Geometry check sheet. Reference: the model listing, model coordinates, mm. Face numbers are marked on the shaded views. A direction names the side the tool comes from. Give positions to 0.01 mm unless a question says otherwise; leave off trailing zeros. Write each loop counter-clockwise with the first axis right and the second up, starting at its lowest first coordinate (ties: lowest second). Pieces come first, ordered by that corner, then holes.
(1) Mould release check, pull along Z, two halves, no side actions. Record for the marked faces 1, 2 and 3: +Z half, -Z half, draft (parallel to the pull), parting line (faces both ways), or undercut.
(2) Cross-section at C-C (z = 3.75). Record the boundary of the cut face in (x, y), and give its area (3 significant figures).
(3) Cross-section at A-A (x = 0). Record the boundary of the cut face in (y, z).
(4) Cross-section at D-D (y = 6.25). Record the boundary of the cut face in (x, z), and give its area (3 significant figures).
(5) Thickness scan on line 1 along X through (y, z) = (2, 4.75); line 2 along Z through (x, y) = (8.75, 3.5); line 3 along X through (y, z) = (5, 4.5). Record the ranges inside material, lowest first.
(6) Cross-section at B-B (z = 0). Record the boundary of the cut face in (x, y).
(7) Tool access check on the marked faces 4 and 5. Record the directions out of +Z, -Z, +X, -X, +Y, -Y that give a thin tool (end or side, any length) a straight path to the whole face; none if there is none.
(8) Depth check by flat-ended pin: P1, Ø3.5, axis at x = 0, z = -9.525, coming from the +Y side; P2, Ø2, axis at y = 3, z = -8.5, coming from the +X side; P3, Ø4, axis at x = -9, y = 6.5, coming from the -Z side. Enter the tip coordinate at first touch or a pass-through.
```python
from build123d import *

# Parameters (mm, degrees)
SKETCH2_R          = 1.4224
CUT_EXTRUDE1_DEPTH = 21.154223776
CIRPATTERN1_COUNT  = 6


with BuildPart() as part:
    # Sketch1 → Revolve1 (revolve)
    with BuildSketch(Plane.XY, mode=Mode.PRIVATE) as revolve1_sk:
        Polygon((2.9972, 0), (12.7, 0), (12.7, 5.08), (6.096, 5.08), (6.096, 9.144), (2.9972, 9.144), align=None)
    revolve(revolve1_sk.sketch.rotate(Axis((0, 0, 0), (0, 1, 0)), 90), axis=Axis((0, 0, 0), (0, 1, 0)))

    # Sketch2 → Cut-Extrude1 (cut, through all)
    with BuildSketch(Plane(origin=(0, 0, 0), x_dir=(1, 0, 0), z_dir=(0, 1, 0))):
        with Locations(Location((0, 9.525, 0), (0, 0, 270))):
            Circle(SKETCH2_R)
    cut_extrude1 = extrude(amount=CUT_EXTRUDE1_DEPTH, mode=Mode.SUBTRACT)

    # CirPattern1: Cut-Extrude1 ×6 about axis
    cirpattern1_axis = Axis((0, 0, 0), (0, 1, 0))
    for i in range(1, CIRPATTERN1_COUNT):
        add(cut_extrude1.rotate(cirpattern1_axis, i * 360 / CIRPATTERN1_COUNT), mode=Mode.SUBTRACT)


solid = part.part
```
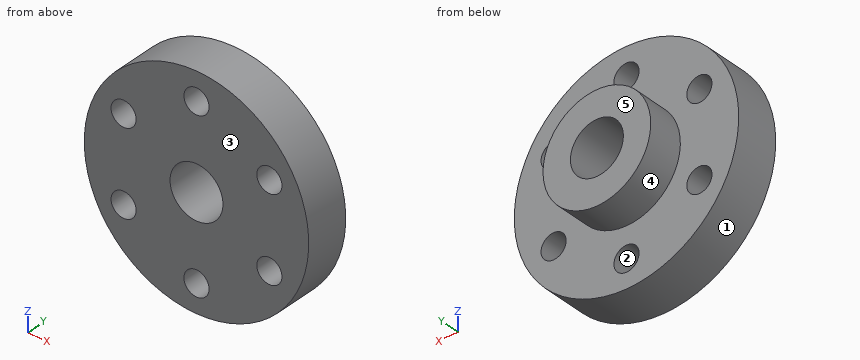
Reply:
1. face 1: parting line
1. face 2: undercut
1. face 3: draft
2. outline: (-12.13, 0) - (-9.25, 0) - (-9.25, 5.08) - (-12.13, 5.08) - close; (-7.25, 0) - (7.25, 0) - (7.25, 5.08) - (4.81, 5.08) - (4.81, 9.14) - (-4.81, 9.14) - (-4.81, 5.08) - (-7.25, 5.08) - close; (9.25, 0) - (12.13, 0) - (12.13, 5.08) - (9.25, 5.08) - close
2. area: 142 mm2
3. outline: (0, -12.7) - (5.08, -12.7) - (5.08, -10.95) - (0, -10.95) - close; (0, -8.1) - (5.08, -8.1) - (5.08, -6.1) - (9.14, -6.1) - (9.14, -3) - (0, -3) - close; (0, 3) - (9.14, 3) - (9.14, 6.1) - (5.08, 6.1) - (5.08, 8.1) - (0, 8.1) - close; (0, 10.95) - (5.08, 10.95) - (5.08, 12.7) - (0, 12.7) - close
4. outline: circle Ø12.19 at (0, 0); hole circle Ø5.99 at (0, 0)
4. area: 88.5 mm2
5. line 1: x = -11.78 to -9.67, -6.83 to 6.83, 9.67 to 11.78
5. line 2: z = -9.2 to -6.09, -3.43 to 3.43, 6.09 to 9.2
5. line 3: x = -11.88 to -9.65, -6.85 to 6.85, 9.65 to 11.88
6. outline: (-12.7, 0) - (-3, 0) - (-3, 9.14) - (-6.1, 9.14) - (-6.1, 5.08) - (-12.7, 5.08) - close; (3, 0) - (12.7, 0) - (12.7, 5.08) - (6.1, 5.08) - (6.1, 9.14) - (3, 9.14) - close
7. face 4: +Y
7. face 5: +Z, -Z, +X, -X, +Y
8. P1: stops at y = 5.08
8. P2: stops at x = 10.25
8. P3: stops at z = -10.18
